Design review of the part shown in the three views and the two pictorial views. Dimensions are in mm from the part's minimum x, y and z. A direction names the side the tool comes from. Give positions to 0.01 mm unless a question says otherwise; leave off trailing zeros. Order: outer loops, then holes, each group sorted by start corner. A loop starts at its lowest first (then second) coordinate and runs counter-clockwise, first axis right, second up.
Item 1: Machinability: for the marked faces 1, 2 and 3, which of the approach directions +Z, -Z, +X, -X, +Y, -Y give a long, thin tool a straight path to every point of the face, cutting with its end or side? Answer none if there is none.
Item 2: Consider section C-C (z = 2.5). Give the boundary of the cut face in (x, y), plus the area to 3 significant figures.
Item 3: Consider section D-D (x = 6.5). Give the boundary of the cut face in (y, z) (3 decimals), plus the area to 3 significant figures.
Item 4: The part is to be moulded in two halves that separate along X. For the marked faces 4, 5 and 6, say which applies: released by +X, released by -X, zero draft, split by the parting line, or undercut.
Item 5: Consider section B-B (x = 4.5). Give the boundary of the cut face in (y, z) (3 decimals), plus the area to 3 significant figures.
Item 6: For P1, Ø1.9, axis at x = 7.025, z = 3.015, coming from the -Y side; P2, Ø3, axis at x = 6.5, y = 9, coming from the -Z side (3 decimals), all flat-tipped, find the tip position at first contact; note any pin that passes through.
Item 7: Consider section A-A (y = 7). Give the boundary of the cut face in (x, z), plus the area to 3 significant figures.
Item 8: For probe 1 along X at (y, z) = (6, 4); probe 2 along Y at (x, z) = (9.75, 5.25); probe 3 along Z at (x, y) = (8.75, 10) (3 decimals), list the stretches that pass through material, from the lowest coordinate up.
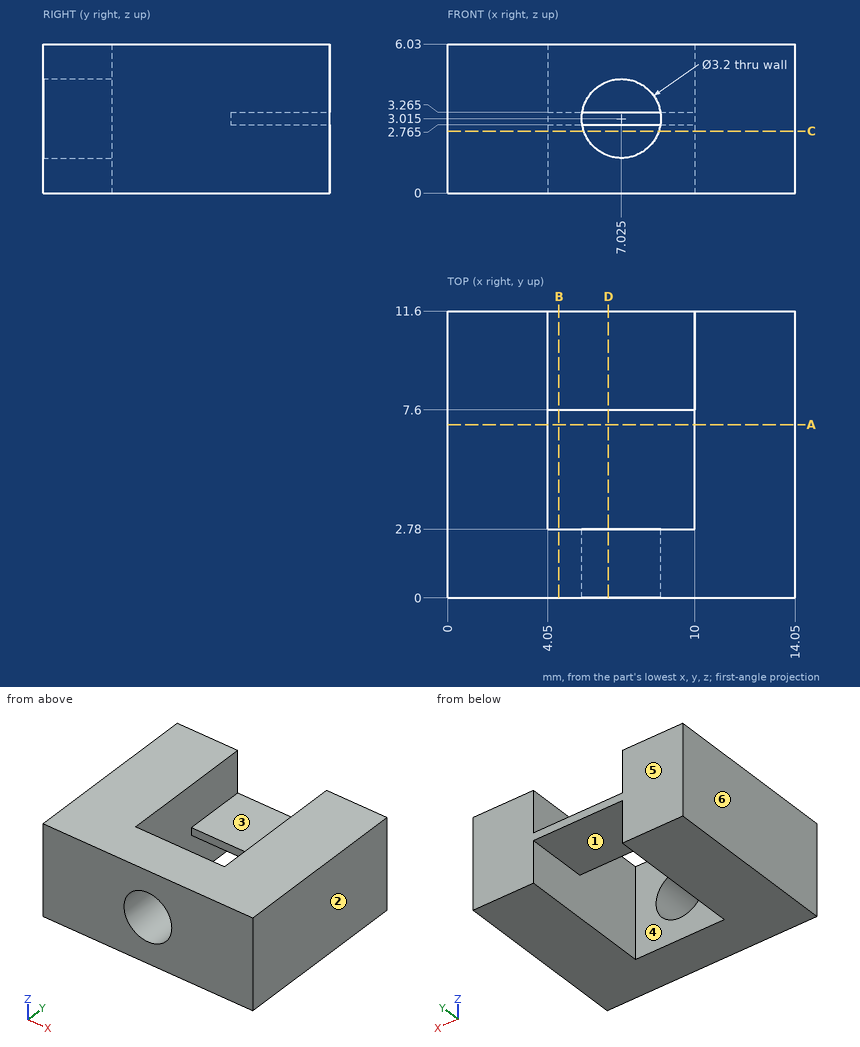
Resolved:
1. face 1: -Z, +Y
1. face 2: +Z, -Z, +X, +Y, -Y
1. face 3: +Z, +Y
2. outline: (0, 0) - (5.51, 0) - (5.51, 2.78) - (4.05, 2.78) - (4.05, 11.6) - (0, 11.6) - close; (8.54, 0) - (14.05, 0) - (14.05, 11.6) - (10, 11.6) - (10, 2.78) - (8.54, 2.78) - close
2. area: 102 mm2
3. outline: (0, 0) - (2.78, 0) - (2.78, 1.504) - (0, 1.504) - close; (0, 4.526) - (2.78, 4.526) - (2.78, 6.03) - (0, 6.03) - close; (7.6, 2.765) - (11.6, 2.765) - (11.6, 3.265) - (7.6, 3.265) - close
3. area: 10.4 mm2
4. face 4: undercut
4. face 5: zero draft
4. face 6: released by -X
5. outline: (0, 0) - (2.78, 0) - (2.78, 6.03) - (0, 6.03) - close; (7.6, 2.765) - (11.6, 2.765) - (11.6, 3.265) - (7.6, 3.265) - close
5. area: 18.8 mm2
6. P1: stops at y = 7.6
6. P2: stops at z = 2.765
7. outline: (0, 0) - (4.05, 0) - (4.05, 6.03) - (0, 6.03) - close; (10, 0) - (14.05, 0) - (14.05, 6.03) - (10, 6.03) - close
7. area: 48.8 mm2
8. probe 1: x = 0 to 4.05, 10 to 14.05
8. probe 2: y = 0 to 2.78
8. probe 3: z = 2.765 to 3.265
